from build123d import *

# Parameters (mm, degrees)
BOX_DEPTH          = 14
TRIANGLE_DEPTH     = 7
SKETCH4_R          = 3
CUT_EXTRUDE1_DEPTH = 33.25405106


with BuildPart() as part:
    # Sketch1 → box (new body)
    with BuildSketch(Plane(origin=(0, 0, 0), x_dir=(1, 0, 0), z_dir=(0, 1, 0))):
        with BuildLine():
            Line((-20, -9), (20, -9))
            ThreePointArc((20, -9), (22.121320344, -8.121320344), (23, -6))
            Line((23, -6), (23, 6))
            ThreePointArc((23, 6), (22.121320344, 8.121320344), (20, 9))
            Line((20, 9), (-20, 9))
            ThreePointArc((-20, 9), (-22.121320344, 8.121320344), (-23, 6))
            Line((-23, 6), (-23, -6))
            ThreePointArc((-23, -6), (-22.121320344, -8.121320344), (-20, -9))
        make_face()
    extrude(amount=BOX_DEPTH)

    # Sketch3 → triangle (add)
    with BuildSketch(Plane.XZ):
        with BuildLine():
            Line((-10, -9), (-2.121320344, -16.878679656))
            ThreePointArc((-2.121320344, -16.878679656), (0, -17.757359313), (2.121320344, -16.878679656))
            Line((2.121320344, -16.878679656), (10, -9))
            Line((10, -9), (-10, -9))
        make_face()
        with BuildLine():
            Line((2.121320344, 16.878679656), (10, 9))
            Line((10, 9), (-10, 9))
            Line((-10, 9), (-2.121320344, 16.878679656))
            ThreePointArc((-2.121320344, 16.878679656), (0, 17.757359313), (2.121320344, 16.878679656))
        make_face()
    extrude(amount=-TRIANGLE_DEPTH)

    # Sketch4 → Cut-Extrude1 (cut, through all)
    with BuildSketch(Plane.XZ):
        with Locations(Location((0, 12.5, 0), (0, 0, 270))):
            Circle(SKETCH4_R)
        with Locations(Location((0, 0, 0), (0, 0, 270))):
            Circle(SKETCH4_R)
        with Locations(Location((0, -12.5, 0), (0, 0, 270))):
            Circle(SKETCH4_R)
    extrude(amount=-CUT_EXTRUDE1_DEPTH, mode=Mode.SUBTRACT)


solid = part.part
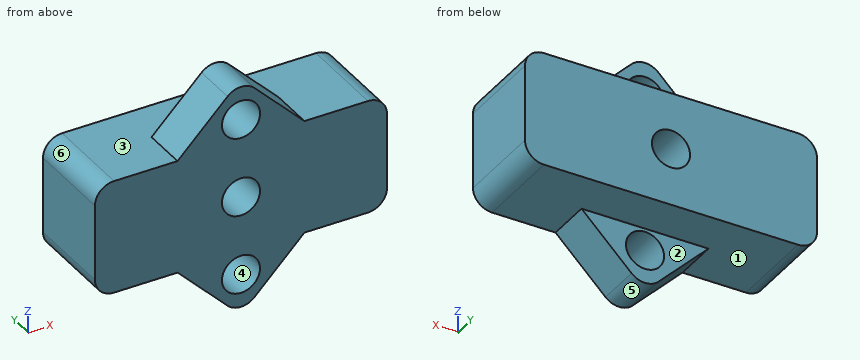
Verification items for the finished model (mm, model axes). Face numbers are marked on the shaded views. A direction names the side the tool comes from. Coordinates: 2 decimals unless noted, no trailing zeros. Order: outer loops, then holes, each group sorted by start corner. A loop starts at its lowest first (then second) coordinate and runs counter-clockwise, first axis right, second up. Notation, with made-up numbers: M 47.25,44.5 L 94.25,44.5 A28 cw 94.25,82.5 Z; hole C 14.5,-21 d6. An arc over 180 degrees is marked long. Write each question's results on one line, items separated by ' | '.
1) Release check for a two-part mould opening along X. For the marked faces 4, 5 and 6 record: pulls with the +X half, pulls with the -X half, needs draft (parallel to the pull), parting line crosses it, or undercut.
Solved:
face 4: undercut | face 5: parting line crosses it | face 6: pulls with the -X half
2) Scan lines: line 1 along X through (y, z) = (7.5, 0); line 2 along X through (y, z) = (1.5, -12.5); line 3 along Z through (x, y) = (-18, 5.75). Record each from-to range of solid material in increasing order. Write a range as [from, to].
Solved:
line 1: x = [-23, -3], [3, 23] | line 2: x = [-6.5, -3], [3, 6.5] | line 3: z = [-9, 9]
3) Section check D-D on y = 5.75. Record the cut outline in (x, z), plus the area to 3 significant figures.
Solved:
outline: M -23,-6 A3 ccw -20,-9 L -10,-9 L -2.12,-16.88 A3 ccw 2.12,-16.88 L 10,-9 L 20,-9 A3 ccw 23,-6 L 23,6 A3 ccw 20,9 L 10,9 L 2.12,16.88 A3 ccw -2.12,16.88 L -10,9 L -20,9 A3 ccw -23,6 Z; hole C 0,-12.5 d6; hole C 0,0 d6; hole C 0,12.5 d6 | area: 932 mm²
4) Access from +Z, -Z, +X, -X, +Y, -Y to the whole of each face (thin tool, end or side, straight path). Record for the marked faces 1, 2 and 3.
Solved:
face 1: -Z, +Y | face 2: -Z, +X, -X, +Y | face 3: +Z, +Y
5) Gauge pin test, flat ends, axial feed: pin 1 Ø4.5 at (x, z) = (-1, -14.5) entering from +Y; pin 2 Ø2 at (x, y) = (-10, 7.5) entering from +Z; pin 3 Ø5 at (x, z) = (0, 12.5) entering from -Y; pin 4 Ø1.5 at (y, z) = (5, -11.5) entering from -X. Record the tip position at first contact, or that the pin passes through.
Solved:
pin 1: stops at y = 7 | pin 2: stops at z = 9.87 | pin 3: passes through | pin 4: stops at x = -8.25
6) Section check C-C on x = 0. Record the cut outline in (y, z), plus the area to 3 significant figures.
Solved:
outline: M 0,-17.76 L 7,-17.76 L 7,-15.5 L 0,-15.5 Z; M 0,-9.5 L 7,-9.5 L 7,-9 L 14,-9 L 14,-3 L 0,-3 Z; M 0,3 L 14,3 L 14,9 L 7,9 L 7,9.5 L 0,9.5 Z; M 0,15.5 L 7,15.5 L 7,17.76 L 0,17.76 Z | area: 207 mm²
7) Section check B-B on z = 12.5. Record the cut outline in (x, y), plus the area to 3 significant figures.
Solved:
outline: M -6.5,0 L -3,0 L -3,7 L -6.5,7 Z; M 3,0 L 6.5,0 L 6.5,7 L 3,7 Z | area: 49.0 mm²
8) Section check A-A on y = 9.25. Record the cut outline in (x, z).
Solved:
outline: M -23,-6 A3 ccw -20,-9 L 20,-9 A3 ccw 23,-6 L 23,6 A3 ccw 20,9 L -20,9 A3 ccw -23,6 Z; hole C 0,0 d6
